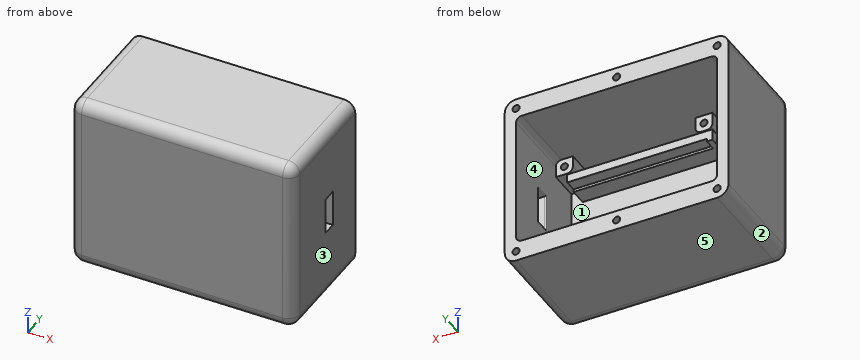
```python
from build123d import *

# Parameters (mm, degrees)
SKETCH1_W                      = 50.0888
SKETCH1_H                      = 39.37
SKETCH1_W_2                    = 45.0088
SKETCH1_H_2                    = 30.48
BOSS_EXTRUDE1_DEPTH            = 23.2918
SKETCH2_W                      = 50.0888
SKETCH2_H                      = 39.37
BOSS_EXTRUDE2_DEPTH            = 2.54
SKETCH3_W                      = 32.512
SKETCH3_H                      = 2.54
BOSS_EXTRUDE3_DEPTH            = 6.5278
F_1_6_1_6_DIAMETER_HOLE1_D     = 1.6
F_1_6_1_6_DIAMETER_HOLE1_DEPTH = 5.08
FILLET1_R                      = 2.54
SKETCH12_W                     = 6.35
SKETCH12_H                     = 7.62
BOSS_EXTRUDE5_DEPTH            = 6.35
F_2_5_2_5_DIAMETER_HOLE2_D     = 2.5
F_2_5_2_5_DIAMETER_HOLE2_DEPTH = 7.62
FILLET2_R                      = 2.54
SKETCH17_W                     = 0.635
SKETCH17_H                     = 2.667
CUT_EXTRUDE3_DEPTH             = 31.242
SKETCH18_W                     = 0.635
SKETCH18_H                     = 2.667
CUT_EXTRUDE5_DEPTH             = 31.242
SKETCH15_W                     = 3.81
SKETCH15_H                     = 3.81
BOSS_EXTRUDE6_DEPTH            = 6.5278
FILLET3_R                      = 1.27
F_1_6_1_6_DIAMETER_HOLE2_D     = 1.6
F_1_6_1_6_DIAMETER_HOLE2_DEPTH = 5.08
CUT_EXTRUDE6_REACH             = 63.109
SKETCH23_W                     = 8.128
SKETCH23_H                     = 3.048
FILLET4_R                      = 0.254
FILLET5_R                      = 1.27


with BuildPart() as part:
    # Sketch1 → Boss-Extrude1 (new body)
    with BuildSketch(Plane(origin=(0, 0, 0), x_dir=(1, 0, 0), z_dir=(0, 1, 0))):
        with Locations((-15.50978333, -6.447590566)):
            Rectangle(SKETCH1_W, SKETCH1_H)
        with Locations((-15.50978333, -6.447590566)):
            Rectangle(SKETCH1_W_2, SKETCH1_H_2, mode=Mode.SUBTRACT)
    extrude(amount=BOSS_EXTRUDE1_DEPTH)

    # Sketch2 → Boss-Extrude2 (add)
    with BuildSketch(Plane.XZ):
        with Locations((-15.50978333, 6.447590566)):
            Rectangle(SKETCH2_W, SKETCH2_H)
    extrude(amount=BOSS_EXTRUDE2_DEPTH)

    # Sketch3 → Boss-Extrude3 (add)
    with BuildSketch(Plane(origin=(0, 0, 0), x_dir=(1, 0, 0), z_dir=(0, 1, 0))):
        with Locations((-11.80138333, 3.458409434)):
            Rectangle(SKETCH3_W, SKETCH3_H)
        with Locations((-11.80138333, -16.353590566)):
            Rectangle(SKETCH3_W, SKETCH3_H)
    extrude(amount=BOSS_EXTRUDE3_DEPTH)

    # Ø1.6 (1.6) Diameter Hole1
    with Locations(Plane(origin=(0, 23.2918, 0), x_dir=(1, 0, 0), z_dir=(0, 1, 0))):
        with Locations((-38.01418333, -23.910090566), (6.99461667, -23.910090566), (6.99461667, 11.014909434), (-38.01418333, 11.014909434), (-15.50978333, 11.014909434), (-15.50978333, -23.910090566)):
            Hole(F_1_6_1_6_DIAMETER_HOLE1_D / 2, depth=F_1_6_1_6_DIAMETER_HOLE1_DEPTH)

    # Fillet1
    fillet1_edges = [part.edges().sort_by_distance(p)[0] for p in [
        (-40.55418333, -2.54, 6.447590566),
        (-15.50978333, -2.54, -13.237409434),
        (9.53461667, -2.54, 6.447590566),
        (-15.50978333, -2.54, 26.132590566),
        (-40.55418333, 10.3759, -13.237409434),
        (9.53461667, 10.3759, -13.237409434),
        (9.53461667, 10.3759, 26.132590566),
        (-40.55418333, 10.3759, 26.132590566),
    ]]
    fillet(fillet1_edges, radius=FILLET1_R)

    # Sketch12 → Boss-Extrude5 (add)
    with BuildSketch(Plane(origin=(-38.01418333, 0, 0), x_dir=(0, 0, -1), z_dir=(1, 0, 0))):
        with Locations((-15.248690566, 6.5278)):
            Rectangle(SKETCH12_W, SKETCH12_H)
        with Locations((2.353509434, 6.5278)):
            Rectangle(SKETCH12_W, SKETCH12_H)
    extrude(amount=BOSS_EXTRUDE5_DEPTH)

    # Ø2.5 (2.5) Diameter Hole2
    with Locations(Plane(origin=(0, 10.3378, 0), x_dir=(1, 0, 0), z_dir=(0, 1, 0))):
        with Locations((-34.83918333, -15.248690566), (-34.83918333, 2.353509434)):
            Hole(F_2_5_2_5_DIAMETER_HOLE2_D / 2, depth=F_2_5_2_5_DIAMETER_HOLE2_DEPTH)

    # Fillet2
    fillet2_edges = [part.edges().sort_by_distance(p)[0] for p in [
        (-31.66418333, 6.5278, 18.423690566),
        (-31.66418333, 6.5278, 12.073690566),
        (-31.66418333, 6.5278, 0.821490566),
        (-31.66418333, 6.5278, -5.528509434),
    ]]
    fillet(fillet2_edges, radius=FILLET2_R)

    # Sketch17 → Cut-Extrude3 (cut)
    with BuildSketch(Plane(origin=(4.45461667, 0, 0), x_dir=(0, 0, -1), z_dir=(1, 0, 0))):
        with Locations((2.505909434, 5.1943)):
            Rectangle(SKETCH17_W, SKETCH17_H)
    extrude(amount=-CUT_EXTRUDE3_DEPTH, mode=Mode.SUBTRACT)

    # Sketch18 → Cut-Extrude5 (cut)
    with BuildSketch(Plane(origin=(4.45461667, 0, 0), x_dir=(0, 0, -1), z_dir=(1, 0, 0))):
        with Locations((-15.401090566, 5.1943)):
            Rectangle(SKETCH18_W, SKETCH18_H)
    extrude(amount=-CUT_EXTRUDE5_DEPTH, mode=Mode.SUBTRACT)

    # Sketch15 → Boss-Extrude6 (add)
    with BuildSketch(Plane(origin=(0, 0, 0), x_dir=(1, 0, 0), z_dir=(0, 1, 0))):
        with Locations((5.08961667, 6.887409434)):
            Rectangle(SKETCH15_W, SKETCH15_H)
        with Locations((-26.15238333, 6.887409434)):
            Rectangle(SKETCH15_W, SKETCH15_H)
        with Locations((-26.15238333, -19.782590566)):
            Rectangle(SKETCH15_W, SKETCH15_H)
        with Locations((5.08961667, -19.782590566)):
            Rectangle(SKETCH15_W, SKETCH15_H)
    extrude(amount=BOSS_EXTRUDE6_DEPTH)

    # Fillet3
    fillet3_edges = [part.edges().sort_by_distance(p)[0] for p in [
        (3.18461667, 3.2639, -4.982409434),
        (-28.05738333, 3.2639, -4.982409434),
        (-24.24738333, 3.2639, -4.982409434),
        (-28.05738333, 3.2639, 17.877590566),
        (-24.24738333, 3.2639, 17.877590566),
        (3.18461667, 3.2639, 17.877590566),
    ]]
    fillet(fillet3_edges, radius=FILLET3_R)

    # Ø1.6 (1.6) Diameter Hole2
    with Locations(Plane(origin=(0, 6.5278, 0), x_dir=(1, 0, 0), z_dir=(0, 1, 0))):
        with Locations((-26.15238333, -19.782590566), (-26.15238333, 6.887409434), (5.08961667, 6.887409434), (5.08961667, -19.782590566)):
            Hole(F_1_6_1_6_DIAMETER_HOLE2_D / 2, depth=F_1_6_1_6_DIAMETER_HOLE2_DEPTH)

    # Sketch23 → Cut-Extrude6 (cut, up to next)
    with BuildSketch(Plane(origin=(9.53461667, 0, 0), x_dir=(0, 0, -1), z_dir=(1, 0, 0)), mode=Mode.PRIVATE) as cut_extrude6_sk1:
        with Locations((-6.447590566, 12.3063)):
            Rectangle(SKETCH23_W, SKETCH23_H)
    cut_extrude6_tool1 = extrude(cut_extrude6_sk1.sketch, amount=-CUT_EXTRUDE6_REACH, mode=Mode.PRIVATE) & part.part
    add(cut_extrude6_tool1.solids().sort_by_distance((9.534617, 12.3063, 6.447591))[0], mode=Mode.SUBTRACT)

    # Fillet4
    fillet4_edges = [part.edges().sort_by_distance(p)[0] for p in [
        (6.99461667, 12.3063, 10.511590566),
        (6.99461667, 13.8303, 6.447590566),
        (6.99461667, 12.3063, 2.383590566),
        (6.99461667, 10.7823, 6.447590566),
    ]]
    fillet(fillet4_edges, radius=FILLET4_R)

    # Fillet5
    fillet5_edges = [part.edges().sort_by_distance(p)[0] for p in [
        (-38.01418333, 11.6459, -8.792409434),
        (-38.01418333, 11.6459, 21.687590566),
        (6.99461667, 14.9098, 21.687590566),
        (6.99461667, 14.9098, -8.792409434),
    ]]
    fillet(fillet5_edges, radius=FILLET5_R)


solid = part.part
```
Model file for the job. Use its own axes, mm. Face numbers are marked on the shaded views. A direction names the side the tool comes from. Round coordinates to 2 decimals unless told otherwise and drop trailing zeros. Write each loop counter-clockwise with the first axis right and the second up, starting at its lowest first coordinate (ties: lowest second). Pieces come first, ordered by that corner, then holes. Notation, with made-up numbers: M 4.5,66.25 L 9.5,66.25 A25 cw 9.5,81.25 Z; hole C 61.5,18 d8. An arc over 180 degrees is marked long. Put each result on its own line as item: value.
Item 1: Cut at C-C (x = -2). List the corners of the cut face in (y, z).
Responses:
outline: M -2.54,-10.7 A2.54 ccw 0,-13.24 L 23.29,-13.24 L 23.29,-8.79 L 0,-8.79 L 0,-4.73 L 6.53,-4.73 L 6.53,-2.82 L 3.86,-2.82 L 3.86,-2.19 L 0,-2.19 L 0,15.08 L 3.86,15.08 L 3.86,15.72 L 6.53,15.72 L 6.53,17.62 L 0,17.62 L 0,21.69 L 23.29,21.69 L 23.29,26.13 L 0,26.13 A2.54 ccw -2.54,23.59 Z
Item 2: Probe L1, parallel to Z at x = -6, y = 6.25; L2, parallel to Z at x = -6, y = 1; L3, parallel to Z at x = -25, y = 8.25. List the from-to ranges inside material, lowest first. Write a range as from..to.
Responses:
L1: -13.24..-8.79, -4.73..-2.82, 15.72..17.62, 21.69..26.13
L2: -13.24..-8.79, -4.73..-2.19, 15.08..17.62, 21.69..26.13
L3: -13.24..-8.79, 21.69..26.13
Item 3: Mould opens along Z. For the marked faces 1, 2 and 3 say: +Z half, -Z half, draft (parallel to the pull), parting line (faces both ways), or undercut.
Responses:
face 1: undercut
face 2: -Z half
face 3: draft
Item 4: Cut at A-A (z = 4). List the corners of the cut face in (x, y).
Responses:
outline: M -40.55,0 A2.54 ccw -38.01,-2.54 L 6.99,-2.54 A2.54 ccw 9.53,0 L 9.53,10.78 L 7.25,10.78 A0.25 ccw 6.99,10.53 L 6.99,0 L -38.01,0 L -38.01,23.29 L -40.55,23.29 Z; M 6.99,14.08 A0.25 ccw 7.25,13.83 L 9.53,13.83 L 9.53,23.29 L 6.99,23.29 Z
Item 5: Cut at D-D (y = 0.75). State how many separate pieces and enclosed holes the cut face has, and give its area (3 significant figures).
Responses:
separate pieces: 3
enclosed holes: 1
area: 816 mm²
Item 6: Flat gauge pins, fed straight in: P1, Ø2, axis at x = -34.84, z = 15.25, coming from the +Y side; P2, Ø1.3, axis at x = -26.5, z = 20, coming from the +Y side; P3, Ø1.3, axis at x = 7, z = 24, coming from the +Y side. Where does each tip first touch, or does it go through?
Responses:
P1: y = 0
P2: y = 6.53
P3: y = 18.21
Item 7: Cut at B-B (y = 17). List the corners of the cut face in (x, z).
Responses:
outline: M -40.55,-10.7 A2.54 ccw -38.01,-13.24 L 6.99,-13.24 A2.54 ccw 9.53,-10.7 L 9.53,23.59 A2.54 ccw 6.99,26.13 L -38.01,26.13 A2.54 ccw -40.55,23.59 Z; hole M -38.01,-7.52 A1.27 ccw -36.74,-8.79 L 5.72,-8.79 A1.27 ccw 6.99,-7.52 L 6.99,20.42 A1.27 ccw 5.72,21.69 L -36.74,21.69 A1.27 ccw -38.01,20.42 Z
Item 8: Tool access for the marked faces 4 and 5: list every direction of +Z, -Z, +X, -X, +Y, -Y with a clear straight run to the whole face (end or side of a thin tool).
Responses:
face 4: +Y
face 5: -Z, +X, -X, +Y, -Y
